Autodesk Inventor part; units mm, degrees
ref_plane "YZ Plane" through (0, 0, 0) normal (1, 0, 0) x (0, 1, 0)
ref_plane "XZ Plane" through (0, 0, 0) normal (0, 1, 0) x (-1, 0, 0)
ref_plane "XY Plane" through (0, 0, 0) normal (0, 0, 1) x (1, 0, 0)
sketch "main" plane through (0, 0, 0) normal (0, 0, 1) x (1, 0, 0)
  circle A0 centre (-31.9195, -99.4713) radius 2.0955
  arc A1 (-38.2695, -99.4713) -> (-33.0376, -105.722) centre (-31.9195, -99.4713) ccw
  arc A2 (-33.0376, -105.722) -> (38.5686, -81.1636) centre (-19.3218, -29.0418) ccw
  line L0 (40.3562, -66.7269) -> (-12.8695, 33.8787)
  line L1 (-12.8695, 33.8787) -> (-12.8695, 119.6037)
  line L2 (-16.0445, 122.7787) -> (-57.3195, 122.7787)
  line L3 (-38.2695, 59.2787) -> (-38.2695, -99.4713)
  arc A3 (38.5686, -81.1636) -> (40.3562, -66.7269) centre (29.1304, -72.6659) ccw
  circle A4 centre (-25.5695, 21.1787) radius 2.0955
  arc A5 (-12.8695, 119.6037) -> (-16.0445, 122.7787) centre (-16.0445, 119.6037) ccw
  circle A6 centre (5.0055, -86.7713) radius 2.0955
  line L4 (-38.2695, 59.2787) -> (-67.8233, 79.8329)
  circle A7 centre (-63.6695, 84.6787) radius 2.1209
  arc A8 (-69.8962, 85.9241) -> (-67.2952, 79.4656) centre (-63.6695, 84.6787) ccw
  circle A9 centre (-57.3195, 116.4287) radius 2.0955
  arc A10 (-57.3195, 122.7787) -> (-63.5462, 117.6741) centre (-57.3195, 116.4287) ccw
  line L5 (-69.8962, 85.9241) -> (-63.5462, 117.6741)
  circle A11 centre (-25.5695, 97.3787) radius 2.0955
  point P0 (-9.1863, -18.3686)
  point P1 (44.2418, -74.0713)
  dimension "d0" = 4.191
  dimension "d1" = 12.7
  dimension "d3" = 4.191
  dimension "d4" = 3.175
  dimension "d5" = 4.191
  dimension "d12" = 4.2418
  dimension "d14" = 4.191
  dimension "d16" = 158.75
  dimension "d17" = 4.191
sketch "Sketch1" plane through (0, 0, 0) normal (1, 0, 0) x (0, 1, 0)
  circle A0 centre (-6.35, -209.55) radius 2.0955
  arc A1 (-12.7, -209.55) -> (-7.4681, -215.8008) centre (-6.35, -209.55) ccw
  arc A2 (-7.4681, -215.8008) -> (64.1381, -191.2423) centre (6.2477, -139.1205) ccw
  line L0 (65.9257, -176.8056) -> (12.7, -76.2)
  line L1 (12.7, -76.2) -> (12.7, 9.525)
  line L2 (9.525, 12.7) -> (-31.75, 12.7)
  line L3 (-12.7, -50.8) -> (-12.7, -209.55)
  arc A3 (64.1381, -191.2423) -> (65.9257, -176.8056) centre (54.7, -182.7446) ccw
  circle A4 centre (0, -88.9) radius 2.0955
  arc A5 (12.7, 9.525) -> (9.525, 12.7) centre (9.525, 9.525) ccw
  circle A6 centre (30.575, -196.85) radius 2.0955
  line L4 (-12.7, -50.8) -> (-42.2538, -30.2459)
  circle A7 centre (-38.1, -25.4) radius 2.1209
  arc A8 (-44.3267, -24.1547) -> (-41.7257, -30.6132) centre (-38.1, -25.4) ccw
  circle A9 centre (-31.75, 6.35) radius 2.0955
  arc A10 (-31.75, 12.7) -> (-37.9767, 7.5953) centre (-31.75, 6.35) ccw
  line L5 (-44.3267, -24.1547) -> (-37.9767, 7.5953)
  circle A11 centre (0, -12.7) radius 2.0955
  point P0 (0, 0)
extrude "Extrusion1" add sketch "Sketch1" along normal blind 1.5875
equation "\"BendRadius\" = Thickness"
equation "\"BendReliefWidth\" = Thickness"
equation "\"BendReliefDepth\" = 0.5 * Thickness"
equation "\"CornerReliefSize\" = 4 * Thickness"
equation "\"MinimumRemnant\" = 2 * Thickness"
equation "\"TransitionRadius\" = BendRadius"
equation "\"JacobiRadiusSize\" = BendRadius"
equation "\"GapSize\" = Thickness"
properties part number "gusset" material "Acetal Resin, White"
Verification items for the finished model (mm, model axes). Give positions to 0.01 mm unless a question says otherwise; leave off trailing zeros. Write each loop counter-clockwise with the first axis right and the second up, starting at its lowest first coordinate (ties: lowest second). Pieces come first, ordered by that corner, then holes. Notation, with made-up numbers: M 52,57.5 L 85,57.5 A20 ccw 85,95.5 Z; hole C 3,-3.5 d6. An arc over 180 degrees is marked long. Use CSV: the item, a comma, the result in double quotes.
1) Cross-section at C-C (y = 0). Enter the section's corners in (x, z).
Final values:
outline,"M 0,-216.77 L 1.59,-216.77 L 1.59,-91 L 0,-91 Z; M 0,-86.8 L 1.59,-86.8 L 1.59,-14.8 L 0,-14.8 Z; M 0,-10.6 L 1.59,-10.6 L 1.59,12.7 L 0,12.7 Z"
2) Cross-section at D-D (z = -12.7). Enter the section's corners in (x, y).
Final values:
outline,"M 0,-42.04 L 1.59,-42.04 L 1.59,-2.1 L 0,-2.1 Z; M 0,2.1 L 1.59,2.1 L 1.59,12.7 L 0,12.7 Z"
3) Cross-section at B-B (z = -88.9). Enter the section's corners in (x, y).
Final values:
outline,"M 0,-12.7 L 1.59,-12.7 L 1.59,-2.1 L 0,-2.1 Z; M 0,2.1 L 1.59,2.1 L 1.59,19.42 L 0,19.42 Z"
4) Material ranges on line 1 along Z through (x, y) = (0.7, 0); line 2 along Z through (x, y) = (0.65, -1); line 3 along Y through (x, z) = (0.65, -209.55), recorded low to high.
Final values:
line 1,"-216.77 to -91, -86.8 to -14.8, -10.6 to 12.7"
line 2,"-216.68 to -90.74, -87.06 to -14.54, -10.86 to 12.7"
line 3,"-12.7 to -8.45, -4.25 to 39.53"
5) Cross-section at A-A (x = 1.15). State how many separate pieces and enclosed holes the cut face has, plus the area to 3 significant figures.
Final values:
separate pieces,"1"
enclosed holes,"6"
area,"11,600 mm²"
6) Release check for a two-part mould opening along Y. For faces 1 (the face through (0.783, -41.196, -8.502)), 2 (the face through (0.783, 32.042, -212.623)), 3 (the face through (0.78, -36.08, -26.04)), 4 (the face through (0.783, 39.685, -127.207)) record: released by +Y, released by -Y, zero draft, split by the parting line, or undercut.
Final values:
face 1,"released by -Y"
face 2,"split by the parting line"
face 3,"undercut"
face 4,"released by +Y"
7) Go/stop test with a flat-tipped pin: pin 1 Ø0.8 at (x, z) = (0.5, -137.5) entering from -Y. Record where the tip stops, or that it passes through.
Final values:
pin 1,"y = -12.7"
